For this review, take the finished solid that the model builds, in its own axes (mm). A direction names the side the tool comes from. Round coordinates to 2 decimals unless told otherwise and drop trailing zeros. Loops run counter-clockwise (first coordinate to the right, second up) from the corner with the lowest first, then second, coordinate; pieces in that order, holes last.
1. To check wall thickness, follow line 1 along Y through (x, z) = (3.75, -3.1); line 2 along X through (y, z) = (29, -2.4); line 3 along X through (y, z) = (15.5, -2.9). State the ranges of each line that lie inside material, in increasing order.
2. Consider section B-B on x = 4.25. State the section outline as (y, z) points.
3. Draft analysis for pull direction Y (two halves, no side actions). For faces 1 (the flat face through (-3.646, 17.109, -1.842)), 2 (the flat face through (6.45, 19.57, -1.84)), 3 (the flat face through (12, 31.1, -1.8)), state which applies: released by +Y, released by -Y, zero draft, split by the parting line, or undercut.
4. Consider section A-A on y = 28.75. State the section outline as (x, z) points, then the cut area to 3 significant figures.
5. Consider section D-D on y = 20. State the section outline as (x, z) points.
6. Clearance check with flat-ended pins moving along their axes: pin 1 Ø1 at (y, z) = (21, -1.5) entering from -X; pin 2 Ø1 at (x, z) = (-2, -2.5) entering from -Y. State where each tip first meets the part, or that it passes through.
7. Tool access review of faces 4 (the flat face through (-2.63, 20.276, -1.842)), 5 (the flat face through (1.189, 16.457, -1.842)), 6 (the flat face through (-4.96, 14.12, -1.84)), 7 (the flat face through (9.082, 29.836, -1.842)), 8 (the flat face through (9.704, 24.914, -1.842)): name each direction out of +Z, -Z, +X, -X, +Y, -Y from which nothing blocks a thin tool from reaching the whole face with its end or side.
8. Consider section C-C on z = -2.4. State the section outline as (x, y) points.
from build123d import *

# Parameters (mm, degrees)
SKETCH_1_R      = 1.3
EXTRUDE_1_DEPTH = 3


with BuildPart() as part:
    # 草图1 → 凸台-拉伸1 (new body)
    with BuildSketch(Plane.XY.offset(-0.362857667)):
        Polygon((6.931968366, 27.685420414), (4.808443123, 29.808337985), (-3.675778765, 21.321687543), (-1.554532399, 19.201048196), (-5.797509256, 14.956856814), (-4.099819599, 13.25965297), (0.142530428, 17.503217343), (2.264294404, 15.382060533), (10.749072595, 23.869267436), (8.629080401, 25.98865297), (12.870428791, 30.231215419), (11.173246227, 31.927912314), align=None)
        with Locations((3.536567574, 22.593983824)):
            Circle(SKETCH_1_R, mode=Mode.SUBTRACT)
    extrude(amount=-EXTRUDE_1_DEPTH)


solid = part.part
Resolved:
1. line 1: y = 16.87 to 21.31, 23.88 to 28.75
1. line 2: x = 4 to 5.62, 8.25 to 11.64
1. line 3: x = -5.25 to -1.86, 2.15 to 2.38
2. outline: (17.37, -3.36) - (21.51, -3.36) - (21.51, -0.36) - (17.37, -0.36) - close; (23.68, -3.36) - (29.25, -3.36) - (29.25, -0.36) - (23.68, -0.36) - close
3. face 1: undercut
3. face 2: released by -Y
3. face 3: released by +Y
4. outline: (3.75, -3.36) - (5.87, -3.36) - (5.87, -0.36) - (3.75, -0.36) - close; (8, -3.36) - (11.39, -3.36) - (11.39, -0.36) - (8, -0.36) - close
4. area: 16.5 mm2
5. outline: (-2.35, -3.36) - (6.88, -3.36) - (6.88, -0.36) - (-2.35, -0.36) - close
6. pin 1: stops at x = -3.68
6. pin 2: stops at y = 14.86
7. face 4: +Z, -Z, -X
7. face 5: +Z, -Z, -Y
7. face 6: +Z, -Z, -X, -Y
7. face 7: +Z, -Z, +Y
7. face 8: +Z, -Z, +X
8. outline: (-5.8, 14.96) - (-4.1, 13.26) - (0.14, 17.5) - (2.26, 15.38) - (10.75, 23.87) - (8.63, 25.99) - (12.87, 30.23) - (11.17, 31.93) - (6.93, 27.69) - (4.81, 29.81) - (-3.68, 21.32) - (-1.55, 19.2) - close; hole circle Ø2.6 at (3.54, 22.59)
